```python
from build123d import *

# Parameters (mm, degrees)
F0_R     = 2.55
F0_R_2   = 0.4
F1_DEPTH = 1.5
F0_R_3   = 3.05
F2_DEPTH = 1.75


with BuildPart() as f1:
    # F0 (on Top) → F1 (new body, symmetric)
    with BuildSketch(Plane.XY):
        Circle(F0_R)
        Polygon((0.016979, -1.683443), (-0.539635, -1.160787), (-0.016979, -0.604173), (0.539635, -1.126829), align=None, mode=Mode.SUBTRACT)
        Polygon((-1.062697, -0.557362), (-1.620059, 0), (-1.062697, 0.557362), (-0.505335, 0), align=None, mode=Mode.SUBTRACT)
        Circle(F0_R_2, mode=Mode.SUBTRACT)
        Polygon((1.1496, -0.591661), (0.55794, 0), (1.1496, 0.591661), (1.741261, 0), align=None, mode=Mode.SUBTRACT)
        Polygon((0, 0.640351), (-0.554009, 1.19436), (0, 1.748368), (0.554009, 1.19436), align=None, mode=Mode.SUBTRACT)
    extrude(amount=F1_DEPTH, both=True)

    # F0 (on Top) → F2 (join, symmetric)
    with BuildSketch(Plane.XY):
        Circle(F0_R_3)
        Circle(F0_R, mode=Mode.SUBTRACT)
    extrude(amount=F2_DEPTH, both=True)


solid = f1.part
```
Input: part model. Units: mm. Frame: model coordinates. A direction names the side the tool comes from. Give positions to 0.01 mm unless a question says otherwise; leave off trailing zeros. Order: outer loops, then holes, each group sorted by start corner. A loop starts at its lowest first (then second) coordinate and runs counter-clockwise, first axis right, second up. Notation, with made-up numbers: M -36.5,88 L -5.5,88 A9 cw -5.5,98 Z; hole C 46,67 d6. An arc over 180 degrees is marked long. One line per question, with ' | ' between items.
1) Section A-A on z = -0.55. Output: boundary loops of the cut face in (x, y), and give its area (3 significant figures).
Filled in:
outline: C 0,0 d6.1; hole M -1.62,0 L -1.06,-0.56 L -0.51,0 L -1.06,0.56 Z; hole M -0.55,1.19 L 0,0.64 L 0.55,1.19 L 0,1.75 Z; hole M -0.54,-1.16 L 0.02,-1.68 L 0.54,-1.13 L -0.02,-0.6 Z; hole C 0,0 d0.8; hole M 0.56,0 L 1.15,-0.59 L 1.74,0 L 1.15,0.59 Z | area: 26.2 mm2
2) Section C-C on x = -1.75. Output: boundary loops of the cut face in (y, z).
Filled in:
outline: M -2.5,-1.75 L -1.85,-1.75 L -1.85,-1.5 L 1.85,-1.5 L 1.85,-1.75 L 2.5,-1.75 L 2.5,1.75 L 1.85,1.75 L 1.85,1.5 L -1.85,1.5 L -1.85,1.75 L -2.5,1.75 Z
3) Section B-B on x = 0.75. Output: boundary loops of the cut face in (y, z), and give its area (3 significant figures).
Filled in:
outline: M -2.96,-1.75 L -2.44,-1.75 L -2.44,-1.5 L -0.19,-1.5 L -0.19,1.5 L -2.44,1.5 L -2.44,1.75 L -2.96,1.75 Z; M 0.19,-1.5 L 2.44,-1.5 L 2.44,-1.75 L 2.96,-1.75 L 2.96,1.75 L 2.44,1.75 L 2.44,1.5 L 0.19,1.5 Z | area: 17.1 mm2
4) Ray query, L1, parallel to Y at x = 0, z = 1.6; L2, parallel to Z at x = 2, y = 1; L3, parallel to Y at x = 1, z = 0.25. Return the intervals inside material, ascending.
Filled in:
L1: y = -3.05 to -2.55, 2.55 to 3.05 | L2: z = -1.5 to 1.5 | L3: y = -2.88 to -0.44, 0.44 to 2.88
5) Draft query along Y for faces 1 (the face through (-3.047, 0.134, 0.024)), 2 (the face through (1, -1, -1.5)), 3 (the face through (2, -2, -1.75)). Return one class per face: pulls with the +Y half, pulls with the -Y half, needs draft (parallel to the pull), parting line crosses it, or undercut.
Filled in:
face 1: parting line crosses it | face 2: undercut | face 3: needs draft
6) Section D-D on y = -2. Output: boundary loops of the cut face in (x, z), and give its area (3 significant figures).
Filled in:
outline: M -2.3,-1.75 L -1.58,-1.75 L -1.58,-1.5 L 1.58,-1.5 L 1.58,-1.75 L 2.3,-1.75 L 2.3,1.75 L 1.58,1.75 L 1.58,1.5 L -1.58,1.5 L -1.58,1.75 L -2.3,1.75 Z | area: 14.5 mm2
7) Access query for faces 4 (the face through (1, -1, 1.5)), 5 (the face through (2, -2, 1.75)). Directions: +Z, -Z, +X, -X, +Y, -Y. A direction counts if a zero-diameter tool reaches every point of the face in a straight line with its end or side. Return the directions, or none.
Filled in:
face 4: +Z | face 5: +Z, +X, -X, +Y, -Y
